Autodesk Inventor part; units mm, degrees
ref_plane "Work Plane1" through (20, 0, 0) normal (1, 0, 0) x (0, 1, 0)
ref_plane "XZ Plane" through (0, 0, 0) normal (0, 1, 0) x (-1, 0, 0)
ref_plane "XY Plane" through (0, 0, 0) normal (0, 0, 1) x (1, 0, 0)
sketch "Sketch1" plane through (0, 0, 0) normal (1, 0, 0) x (0, 1, 0)
  line L0 (12, 4.5) -> (12, 8.5)
  line L1 (2.8235, 2) -> (12, 8.5)
  line L2 (17.8235, -12.625) -> (2.8235, -2)
  line L3 (0, 0) -> (0, 2)
  line L4 (0, 2) -> (2.8235, 2)
  line L5 (0, 0) -> (0, -2)
  line L6 (0, -2) -> (2.8235, -2)
  line L7 (12, 4.5) -> (5.6471, 0)
  line L8 (17.8235, -12.625) -> (17.8235, -8.625)
  line L9 (5.6471, 0) -> (17.8235, -8.625)
  dimension "d7" = 12
  dimension "d9" = 2
  dimension "d10" = 2
  dimension "d12" = 4
  dimension "d26" = 9.1765
  dimension "d27" = 6.3529
  dimension "d53" = 70.622
  dimension "d55" = 144.689
  dimension "d56" = 15
ref_plane "Work Plane1" through (20, 0, 0) normal (1, 0, 0) x (0, 1, 0)
sketch "Sketch2" plane through (20, 0, 0) normal (1, 0, 0) x (0, 1, 0)
  line L0 (12, 4.5) -> (12, 8.5)
  line L1 (12, 4.5) -> (5.6471, 0)
  line L2 (2.8235, 2) -> (12, 8.5)
  line L3 (17.8235, -12.625) -> (2.8235, -2)
  line L4 (0, 2) -> (2.8235, 2)
  line L5 (0, 0) -> (0, 2)
  line L6 (0, 0) -> (0, -2)
  line L7 (0, -2) -> (2.8235, -2)
  line L8 (5.75, 0) -> (12, 4.5)
  line L9 (17.8235, -12.625) -> (2.8235, -2)
  line L10 (0, -2) -> (2.8235, -2)
  line L11 (0, -2) -> (0, 2)
  line L12 (0, 2) -> (2.8235, 2)
  line L13 (2.8235, 2) -> (12, 8.5)
  line L14 (12, 8.5) -> (12, 4.5)
  line L15 (17.8235, -12.625) -> (17.8235, -8.625)
  line L16 (17.8235, -8.625) -> (5.75, 0)
  dimension "d19" = 0.1029
  dimension "d57" = 4
  dimension "d58" = 71.295
loft "Loft1" add profiles "Sketch1", "Sketch2"
fillet "Fillet1" radius 1 1 edges at (10, 5.6985, 0)
sketch "Sketch3" plane through (20, 0, -2) normal (1, 0, 0) x (0, 0, -1)
  line L0 (-4, 2.8235) -> (-10.5, 12)
  line L1 (-4, 2.8235) -> (0, 2.8235)
  line L2 (0, 2.8235) -> (0, -28.6765)
  line L3 (0, -28.6765) -> (-4, -28.6765)
  line L4 (-4, -24.6765) -> (-4, 2.8235)
  line L5 (0, -28.6765) -> (-15, -28.6765)
  line L6 (-15, -28.6765) -> (-15, -24.6765)
  line L7 (-15, -24.6765) -> (-4, -24.6765)
  line L8 (0, -24.6765) -> (0, -28.6765)
  point P0 (-2, 0)
  dimension "d35" = 31.5
  dimension "d36" = 4
  dimension "d37" = 15
  dimension "d38" = 4
  dimension "d39" = 11
extrude "Extrusion2" add sketch "Sketch3" against normal up to surface (20 mm away)
sketch "Sketch4" plane through (20, -28.6765, -2) normal (0, -1, 0) x (1, 0, 0)
  line L0 (0, 15) -> (-20, 15)
  line L1 (-20, 0) -> (-20, 15)
  line L2 (0, 0) -> (0, 15)
  circle A0 centre (-14, 10) radius 0.7925
  circle A1 centre (-6, 10) radius 0.7925
  point P0 (-20, 2)
  dimension "d44" = 5
  dimension "d45" = 6
  dimension "d46" = 6
  dimension "d48" = 5
  dimension "d49" = 1.585
  dimension "d50" = 1.585
extrude "Extrusion3" cut sketch "Sketch4" against normal blind 10
equation "\"d19\" = d15"
equation "\"d50\" = d49"
properties part number "stopper"
Can you work these out from the model? Positions are in its coordinate system, mm. A direction names the side the tool comes from. Give positions to 0.01 mm unless a question says otherwise; leave off trailing zeros. Loops run counter-clockwise (first coordinate to the right, second up) from the corner with the lowest first, then second, coordinate; pieces in that order, holes last. Notation, with made-up numbers: (82, 84.25) -> (132, 84.25) arc R29 cw to (132, 112.25) -> close; hole circle Ø2 at (-32.75, 10.5). An arc over 180 degrees is marked (long way). Write item = value, one per line.
1) For faces 1 (the flat face through (10, -24.676, 8)), 2 (the flat face through (10, -27, 13)), 3 (the cylindrical face through (13.42, -26.7, 8.54)), which set-ups out of +Z, -Z, +X, -X, +Y, -Y let a thin tool reach every point of the face, with its end or its side?
Check result:
face_1 = +Z, +X, -X
face_2 = +Z, +X, -X, +Y, -Y
face_3 = -Y
2) Suppose I cut it at C-C on z = -10.25. Write out the boundary of the cut face in (x, y).
Check result:
outline = (0, 14.47) -> (20, 14.47) -> (20, 17.82) -> (0, 17.82) -> close
3) Suppose I cut it at B-B on y = -8.5. Write out the boundary of the cut face in (x, z), then the cut area to 3 significant figures.
Check result:
outline = (0, -2) -> (20, -2) -> (20, 2) -> (0, 2) -> close
area = 80.0 mm2
4) Will these pins go through, and if not, where does the flat tip stop? pin 1 (6 mm diameter, centred on x = 14.5, y = -8.5, fed in from +Z); pin 2 (2 mm diameter, centred on x = 10, y = -5, fed in from -Z); pin 3 (1.2 mm diameter, centred on x = 13, z = 6, fed in from +Y); pin 4 (12 mm diameter, centred on y = -23.5, z = 6, fed in from +X).
Check result:
pin_1 = 2
pin_2 = -2
pin_3 = 12
pin_4 = 20
5) Suppose I cut it at A-A on z = 8. Write out the boundary of the cut face in (x, y).
Check result:
outline = (0, -28.68) -> (5.21, -28.68) -> (5.21, -24.68) -> (0, -24.68) -> close; (0, 11.29) -> (20, 11.29) -> (20, 12) -> (0, 12) -> close; (6.79, -28.68) -> (13.21, -28.68) -> (13.21, -24.68) -> (6.79, -24.68) -> close; (14.79, -28.68) -> (20, -28.68) -> (20, -24.68) -> (14.79, -24.68) -> close
6) Thinking about a two-plate mould opening in Z: for faces 4 (the flat face through (10, 12, 6)), 5 (the flat face through (10, -13, -2)), 6 (the flat face through (10.14, 7.48, 5.3)), 7 (the cylindrical face through (5.42, -26.7, 8.54)), which applies, released by +Z, released by -Z, zero draft, split by the parting line, or undercut?
Check result:
face_4 = zero draft
face_5 = released by -Z
face_6 = released by +Z
face_7 = undercut
7) I need wall thicknesses on L1, parallel to Z at x = 14, y = -25.6; L2, parallel to Y at x = 11.5, z = 7; L3, parallel to Z at x = 2, y = -15. Which ranges of each line are inside material? Lowest first, please. Write a range as from..to.
Check result:
L1 = -2..7.21, 8.79..13
L2 = -28.68..-24.68, 9.88..12
L3 = -2..2
